Geometry: final body of the model. Coordinates: model frame, mm. A direction names the side the tool comes from. Coordinates: 2 decimals unless noted, no trailing zeros. Write each loop counter-clockwise with the first axis right and the second up, starting at its lowest first coordinate (ties: lowest second). Pieces come first, ordered by that corner, then holes. Notation, with made-up numbers: (89.5, -23) -> (136.5, -23) arc R18 cw to (136.5, -1) -> close; hole circle Ø2 at (43, 23.5). An arc over 180 degrees is marked (long way). One line per item, written item: value.
```python
from build123d import *

# Parameters (mm, degrees)
BOSS_EXTRUDE1_DEPTH = 15
SKETCH2_R           = 10
BOSS_EXTRUDE2_DEPTH = 90


with BuildPart() as part:
    # Sketch1 → Boss-Extrude1 (new body)
    with BuildSketch(Plane.XY):
        Polygon((-20.207259422, 0), (-10.103629711, -17.5), (10.103629711, -17.5), (20.207259422, 0), (10.103629711, 17.5), (-10.103629711, 17.5), align=None)
    extrude(amount=BOSS_EXTRUDE1_DEPTH)

    # Sketch2 → Boss-Extrude2 (add)
    with BuildSketch(Plane.XY.offset(15)):
        Circle(SKETCH2_R)
    extrude(amount=BOSS_EXTRUDE2_DEPTH)

    # Sketch3 → Cut-Revolve2 (revolve, cut)
    with BuildSketch(Plane(origin=(0, 0, 0), x_dir=(1, 0, 0), z_dir=(0, 1, 0))):
        with BuildLine():
            Line((18.207259422, 0), (20.207259422, 0))
            Line((20.207259422, 0), (20.207259422, -2))
            ThreePointArc((20.207259422, -2), (19.621472984, -0.585786438), (18.207259422, 0))
        make_face()
    revolve(axis=Axis((0, 0, 105), (0, 0, -1)), mode=Mode.SUBTRACT)


solid = part.part
```
(1) Section A-A (x = 0). Return the cut outline in (y, z), then the cut area to 4 significant figures.
Responses:
outline: (-17.5, 0) -> (17.5, 0) -> (17.5, 15) -> (10, 15) -> (10, 105) -> (-10, 105) -> (-10, 15) -> (-17.5, 15) -> close
area: 2,325 mm2
(2) Line query: line 1 (Z direction, x = 13, y = -8.5); line 2 (Y direction, x = 3.5, z = 42.5); line 3 (X direction, y = -4.5, z = 80.5). Output: solid intervals per line, ascending. Write a range as [from, to].
Responses:
line 1: z = [0, 15]
line 2: y = [-9.37, 9.37]
line 3: x = [-8.93, 8.93]
(3) Section D-D (x = -16). Return the cut outline in (y, z).
Responses:
outline: (-7.29, 0) -> (7.29, 0) -> (7.29, 15) -> (-7.29, 15) -> close
(4) Reachability of faces 1 (the cylindrical face through (-2.17, -9.76, 59.37)), 2 (the flat face through (0, -17.5, 7)) from +Z, -Z, +X, -X, +Y, -Y: full face, straight path, thin tool, end or side. Return the list, or none.
Responses:
face 1: +Z
face 2: +Z, -Z, +X, -X, -Y
(5) Section B-B (z = 31.5). Return the cut outline in (x, y).
Responses:
outline: circle Ø20 at (0, 0)
(6) Section C-C (y = 11). Return the cut outline in (x, z), then the cut area to 3 significant figures.
Responses:
outline: (-13.86, 0) -> (13.86, 0) -> (13.86, 15) -> (-13.86, 15) -> close
area: 416 mm2
(7) First-contact query: pin 1 (1 mm diameter, centred on y = -3.5, z = 80.5, fed in from -X); pin 2 (1 mm diameter, centred on y = 9, z = 58, fed in from -X); pin 3 (5 mm diameter, centred on x = 7, z = 45, fed in from -Y). Flat tips, straight axial feed; report the tip coordinate or a pass-through.
Responses:
pin 1: stops at x = -9.54
pin 2: stops at x = -5.27
pin 3: stops at y = -8.93
